Could you check a few things on this drawing? It's one solid part, dimensions in mm from its lowest x, y, z. Give positions to 0.01 mm unless a question says otherwise; leave off trailing zeros. Order: outer loops, then holes, each group sorted by start corner. A loop starts at its lowest first (then second) coordinate and runs counter-clockwise, first axis right, second up.
(1) Imagine slicing it at C-C, the plane z = 1.55. Write out the boundary of the cut face in (x, y).
(2) Imagine slicing it at A-A, the plane x = 8. Write out the boundary of the cut face in (y, z), then the cut area to 3 significant figures.
(3) If I drill on probe 1 along Y at (x, z) = (8, 1); probe 2 along X at (y, z) = (53.5, 0.95); probe 3 along X at (y, z) = (51.5, 0.8), over which ranges is the centre line in solid material (lowest first)?
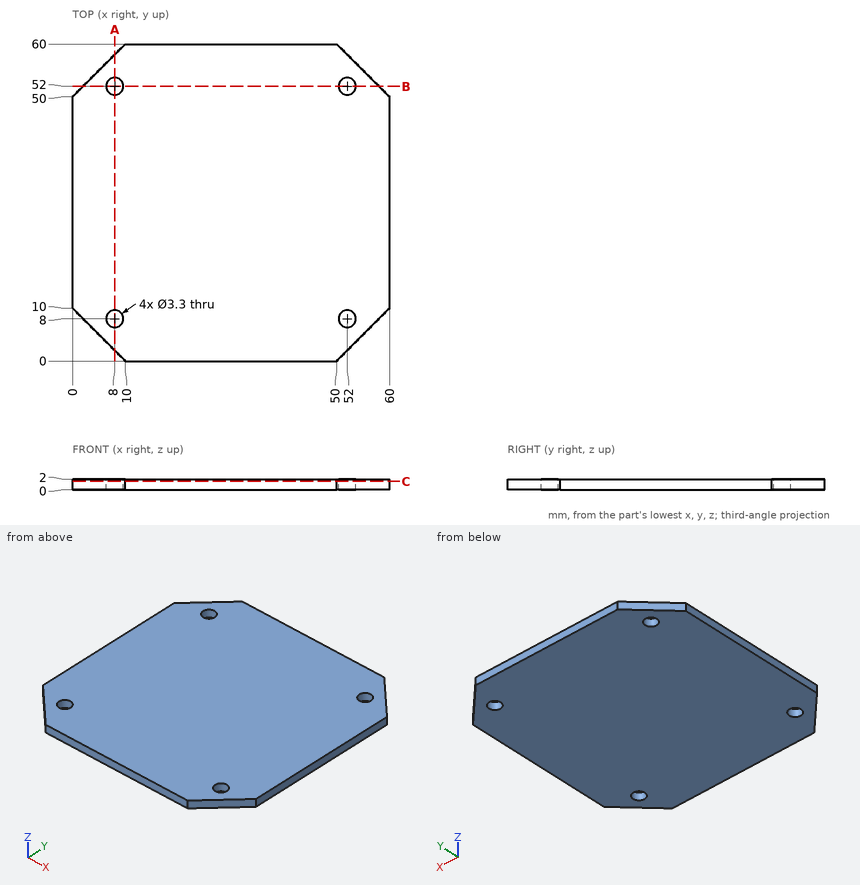
Answer block:
1. outline: (0, 10) - (10, 0) - (50, 0) - (60, 10) - (60, 50) - (50, 60) - (10, 60) - (0, 50) - close; hole circle Ø3.3 at (8, 8); hole circle Ø3.3 at (8, 52); hole circle Ø3.3 at (52, 8); hole circle Ø3.3 at (52, 52)
2. outline: (2, 0) - (6.35, 0) - (6.35, 2) - (2, 2) - close; (9.65, 0) - (50.35, 0) - (50.35, 2) - (9.65, 2) - close; (53.65, 0) - (58, 0) - (58, 2) - (53.65, 2) - close
2. area: 98.8 mm2
3. probe 1: y = 2 to 6.35, 9.65 to 50.35, 53.65 to 58
3. probe 2: x = 3.5 to 7.31, 8.69 to 51.31, 52.69 to 56.5
3. probe 3: x = 1.5 to 6.43, 9.57 to 50.43, 53.57 to 58.5
